Design review of the part shown in the three views and the two pictorial views. Dimensions are in mm from the part's minimum x, y and z. Give positions to 0.01 mm unless a question says otherwise; leave off trailing zeros. Write each loop counter-clockwise with the first axis right and the second up, starting at its lowest first coordinate (ties: lowest second). Pieces come first, ordered by that corner, then holes.
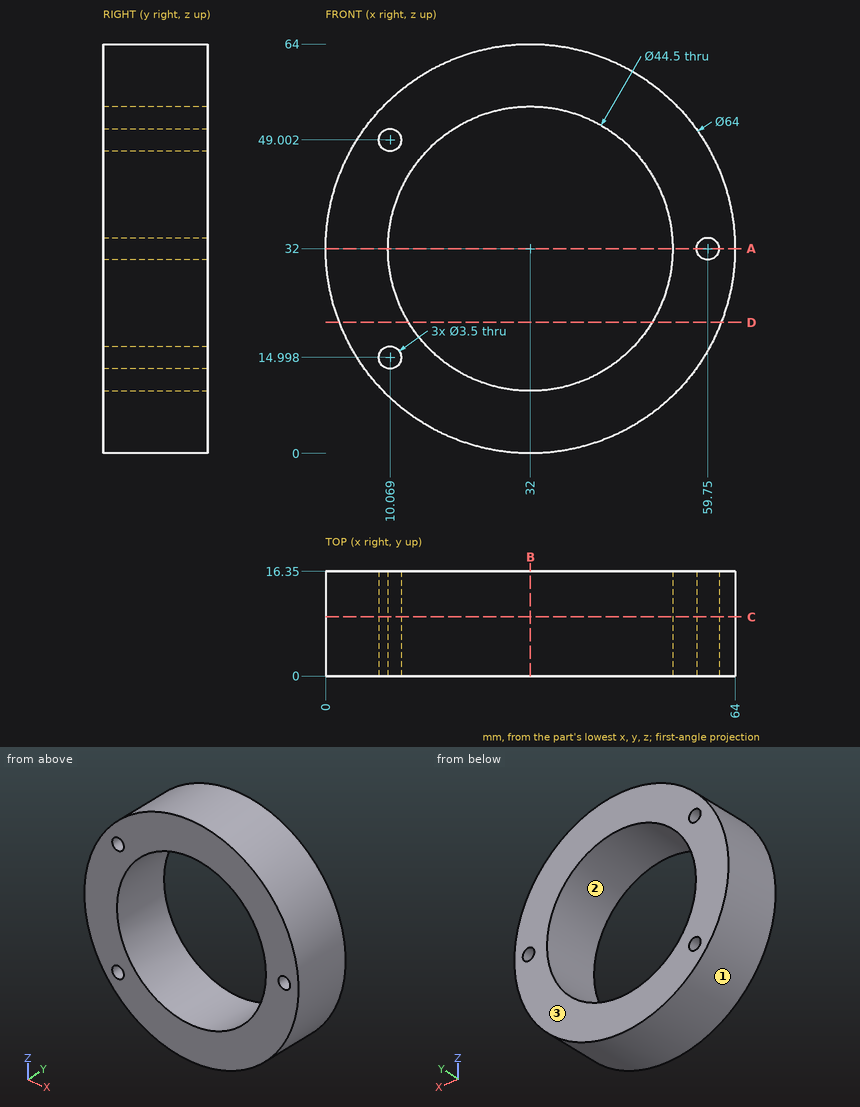
(1) Consider section D-D, the plane z = 20.5. Give the boundary of the cut face in (x, y), then the cut area to 3 significant figures.
Resolved:
outline: (2.14, 0) - (12.95, 0) - (12.95, 16.35) - (2.14, 16.35) - close; (51.05, 0) - (61.86, 0) - (61.86, 16.35) - (51.05, 16.35) - close
area: 354 mm2
(2) To check wall thickness, follow L1, parallel to X at y = 13, z = 32; L2, parallel to X at y = 2.75, z = 14 (1 decimal); L3, parallel to Z at x = 55, y = 11.75. State the ranges of each line that lie inside material, in increasing order.
Resolved:
L1: x = 0 to 9.75, 54.25 to 58, 61.5 to 64
L2: x = 5.5 to 8.6, 11.5 to 18.9, 45.1 to 58.5
L3: z = 9.75 to 54.25
(3) Clearance check with flat-ended pins moving along their axes: P1, Ø2, axis at y = 14.5, z = 7, coming from the +X side (1 decimal); P2, Ø4, axis at x = 15, z = 43.5, coming from the -Y side; P3, Ø5, axis at y = 2, z = 16, coming from the +X side. State where each tip first meets the part, or that it passes through.
Resolved:
P1: stops at x = 53.2
P2: stops at y = 0
P3: stops at x = 61.01
(4) Consider section C-C, the plane y = 9.25. Give the boundary of the cut face in (x, z), then the cut area to 3 significant figures.
Resolved:
outline: circle Ø64 at (32, 32); hole circle Ø3.5 at (10.07, 15); hole circle Ø3.5 at (10.07, 49); hole circle Ø44.5 at (32, 32); hole circle Ø3.5 at (59.75, 32)
area: 1,630 mm2
(5) Consider section A-A, the plane z = 32. Give the boundary of the cut face in (x, y).
Resolved:
outline: (0, 0) - (9.75, 0) - (9.75, 16.35) - (0, 16.35) - close; (54.25, 0) - (58, 0) - (58, 16.35) - (54.25, 16.35) - close; (61.5, 0) - (64, 0) - (64, 16.35) - (61.5, 16.35) - close
(6) Mouldability with a two-part tool opening along Z and no side actions: class the marked faces 1, 2 and 3 as pulls with the +Z half, pulls with the -Z half, needs draft (parallel to the pull), parting line crosses it, or undercut.
Resolved:
face 1: parting line crosses it
face 2: undercut
face 3: needs draft
(7) Consider section B-B, the plane x = 32. Give the boundary of the cut face in (y, z).
Resolved:
outline: (0, 0) - (16.35, 0) - (16.35, 9.75) - (0, 9.75) - close; (0, 54.25) - (16.35, 54.25) - (16.35, 64) - (0, 64) - close
